For this review, take the finished solid that the model builds, in its own axes (mm). Face numbers are marked on the shaded views. A direction names the side the tool comes from. Give positions to 0.01 mm unless a question says otherwise; leave off trailing zeros. Loops run counter-clockwise (first coordinate to the right, second up) from the corner with the lowest first, then second, coordinate; pieces in that order, holes last.
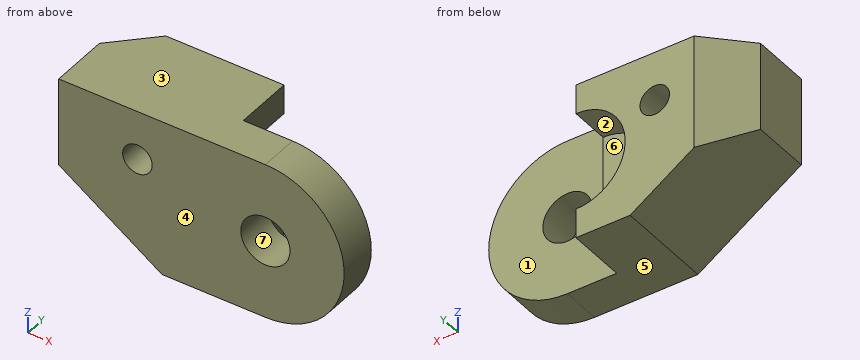
```python
from build123d import *

# Parameters (mm, degrees)
F0_R     = 9.525
F0_R_2   = 15.875
F1_DEPTH = 31.75
F2_W     = 50.8
F2_H     = 38.1
F2_W_2   = 31.75
F3_DEPTH = 127
F5_DEPTH = 25.4


with BuildPart() as f1:
    # F0 (on Front) → F1 (new body, symmetric)
    with BuildSketch(Plane.XZ):
        with BuildLine():
            Line((-66.675, -50.8), (0, -50.8))
            ThreePointArc((0, -50.8), (50.8, 0), (0, 50.8))
            Line((0, 50.8), (-133.35, 50.8))
            Line((-133.35, 50.8), (-133.35, -6.35))
            Line((-133.35, -6.35), (-66.675, -50.8))
        make_face()
        with Locations((-82.55, 19.05)):
            Circle(F0_R, mode=Mode.SUBTRACT)
        Circle(F0_R_2, mode=Mode.SUBTRACT)
    extrude(amount=F1_DEPTH, both=True)

    # F2 (on face) → F3 (cut)
    with BuildSketch(Plane.XY.offset(50.8)):
        Polygon((-133.35, 6.35), (-107.95, 31.75), (-133.35, 31.75), align=None)
        with Locations((25.4, 12.7)):
            Rectangle(F2_W, F2_H)
        with Locations((-15.875, 12.7)):
            Rectangle(F2_W_2, F2_H)
    extrude(amount=-F3_DEPTH, mode=Mode.SUBTRACT)

    # F4 (on face) → F5 (cut)
    with BuildSketch(Plane(origin=(0, 31.75, 0), x_dir=(-1, 0, 0), z_dir=(0, 1, 0))):
        with BuildLine():
            Line((31.75, 0), (31.75, -31.75))
            ThreePointArc((31.75, -31.75), (63.5, 0), (31.75, 31.75))
            Line((31.75, 31.75), (31.75, 0))
        make_face()
    extrude(amount=-F5_DEPTH, mode=Mode.SUBTRACT)


solid = f1.part
```
Item 1: The part is to be moulded in two halves that separate along Z. For the marked faces 4, 5, 6 and 7, say which applies: released by +Z, released by -Z, zero draft, split by the parting line, or undercut.
Answer:
face 4: zero draft
face 5: released by -Z
face 6: undercut
face 7: undercut
Item 2: Take a section at C-C on y = -24. Give the boundary of the cut face in (x, z) (3 decimals), and give its area (3 significant figures).
Answer:
outline: (-133.35, -6.35) - (-66.675, -50.8) - (0, -50.8) arc R50.8 ccw to (0, 50.8) - (-133.35, 50.8) - close; hole circle Ø19.05 at (-82.55, 19.05); hole circle Ø31.75 at (0, 0)
area: 15,000 mm2
Item 3: For L1, parallel to Y at x = 20.5, z = 9; L2, parallel to Z at x = -9, y = -16; L3, parallel to Z at x = -79, y = 15, list the stretches that pass through material, from the lowest coordinate up.
Answer:
L1: y = -31.75 to -6.35
L2: z = -50.8 to -13.08, 13.08 to 50.8
L3: z = -42.58 to 10.21, 27.89 to 50.8
Item 4: Take a section at D-D on y = 17. Give the boundary of the cut face in (x, z) (3 decimals), and give its area (3 significant figures).
Answer:
outline: (-122.7, -13.45) - (-66.675, -50.8) - (-31.75, -50.8) - (-31.75, -31.75) arc R31.75 cw to (-31.75, 31.75) - (-31.75, 50.8) - (-122.7, 50.8) - close; hole circle Ø19.05 at (-82.55, 19.05)
area: 6,330 mm2
Item 5: Tool access review of the marked faces 1, 2 and 3: name each direction out of +Z, -Z, +X, -X, +Y, -Y from which nothing blocks a thin tool from reaching the whole face with its end or side.
Answer:
face 1: +Z, -Z, +X, +Y
face 2: +X, +Y
face 3: +Z, +X, -X, +Y, -Y
Item 6: Take a section at B-B on x = 6. Give the boundary of the cut face in (y, z), and give its area (3 significant figures).
Answer:
outline: (-31.75, -50.44) - (-6.35, -50.44) - (-6.35, -14.7) - (-31.75, -14.7) - close; (-31.75, 14.7) - (-6.35, 14.7) - (-6.35, 50.44) - (-31.75, 50.44) - close
area: 1,820 mm2
Item 7: Clearance check with flat-ended pins moving along their axes: pin 1 Ø8 at (x, z) = (-2, 30) entering from +Y; pin 2 Ø3 at (x, y) = (-107.5, -7) entering from -Z; pin 3 Ø16 at (x, z) = (-49, -5) entering from +Y; pin 4 Ø22 at (x, z) = (-82.55, 19.05) entering from -Y. State where each tip first meets the part, or that it passes through.
Answer:
pin 1: stops at y = -6.35
pin 2: stops at z = -24.58
pin 3: stops at y = 6.35
pin 4: stops at y = -31.75
Item 8: Take a section at A-A on z = 0. Give the boundary of the cut face in (x, y) (3 decimals), and give its area (3 significant figures).
Answer:
outline: (-133.35, -31.75) - (-15.875, -31.75) - (-15.875, -6.35) - (-31.75, -6.35) - (-31.75, 6.35) - (-63.5, 6.35) - (-63.5, 31.75) - (-107.95, 31.75) - (-133.35, 6.35) - close; (15.875, -31.75) - (50.8, -31.75) - (50.8, -6.35) - (15.875, -6.35) - close
area: 6,610 mm2
